Geometry: final body of the model. Coordinates: model frame, mm. Face numbers are marked on the shaded views. A direction names the side the tool comes from. Coordinates: 2 decimals unless noted, no trailing zeros. Order: outer loops, then holes, each group sorted by start corner. A loop starts at its lowest first (then second) coordinate and runs counter-clockwise, first axis right, second up. Notation, with made-up numbers: (-3.75, -26.75) - (28.25, -26.75) arc R11 cw to (28.25, -7.75) - close; hole circle Ø4 at (21.25, 23). An arc over 180 degrees is marked (long way). Use a Markdown table: item, result. Add a question column.
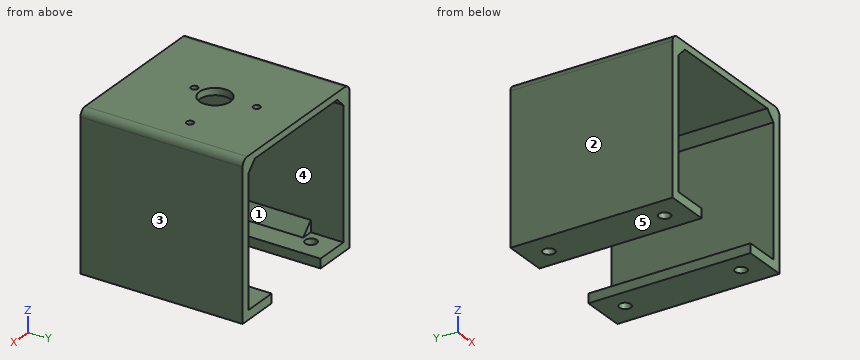
```python
from build123d import *

# Parameters (mm, degrees)
SKETCH1_W                = 70
SKETCH1_H                = 70
BOSS_EXTRUDE2_DEPTH      = 3
SKETCH2_R                = 6.75
SKETCH2_R_2              = 1.5
CUT_EXTRUDE1_DEPTH       = 4
SKETCH3_W                = 64
SKETCH3_H                = 70
BOSS_EXTRUDE3_DEPTH      = 4
SKETCH4_W                = 64
SKETCH4_H                = 70
BOSS_EXTRUDE4_DEPTH      = 4
SKETCH5_W                = 15
SKETCH5_H                = 70
BOSS_EXTRUDE5_DEPTH      = 4
SKETCH6_R                = 2.5
CUT_EXTRUDE2_DEPTH       = 4
BOSS_EXTRUDE6_DEPTH      = 70
BOSS_EXTRUDE7_DEPTH      = 20
BOSS_EXTRUDE7_DEPTH_BACK = 19
FILLET1_R                = 3


with BuildPart() as part:
    # Sketch1 → Boss-Extrude2 (new body)
    with BuildSketch(Plane.XY):
        with Locations((-9.605752423, -0.918004132)):
            Rectangle(SKETCH1_W, SKETCH1_H)
    extrude(amount=BOSS_EXTRUDE2_DEPTH)

    # Sketch2 → Cut-Extrude1 (cut)
    with BuildSketch(Plane.XY.offset(3)):
        with Locations((-9.605752423, -0.918004132)):
            Circle(SKETCH2_R)
        with Locations((-11.293574597, 16.005389627)):
            Circle(SKETCH2_R_2)
        with Locations((11.956425403, 2.581995868)):
            Circle(SKETCH2_R_2)
        with Locations((-11.293574597, -10.84139789)):
            Circle(SKETCH2_R_2)
    extrude(amount=-CUT_EXTRUDE1_DEPTH, mode=Mode.SUBTRACT)

    # Sketch3 → Boss-Extrude3 (add)
    with BuildSketch(Plane(origin=(25.394247577, 0, 0), x_dir=(0, 0, -1), z_dir=(1, 0, 0))):
        with Locations((32, -0.918004132)):
            Rectangle(SKETCH3_W, SKETCH3_H)
    extrude(amount=-BOSS_EXTRUDE3_DEPTH)

    # Sketch4 → Boss-Extrude4 (add)
    with BuildSketch(Plane.ZY.offset(44.605752423)):
        with Locations((-32, -0.918004132)):
            Rectangle(SKETCH4_W, SKETCH4_H)
    extrude(amount=-BOSS_EXTRUDE4_DEPTH)

    # Sketch5 → Boss-Extrude5 (add)
    with BuildSketch(Plane(origin=(0, 0, -64), x_dir=(-1, 0, 0), z_dir=(0, 0, -1))):
        with Locations((-13.894247577, -0.918004132)):
            Rectangle(SKETCH5_W, SKETCH5_H)
        with Locations((33.105752423, -0.918004132)):
            Rectangle(SKETCH5_W, SKETCH5_H)
    extrude(amount=-BOSS_EXTRUDE5_DEPTH)

    # Sketch6 → Cut-Extrude2 (cut)
    with BuildSketch(Plane(origin=(0, 0, -64), x_dir=(-1, 0, 0), z_dir=(0, 0, -1))):
        with Locations((-15.394247577, 24.081995868)):
            Circle(SKETCH6_R)
        with Locations((-15.394247577, -25.918004132)):
            Circle(SKETCH6_R)
        with Locations((34.605752423, 24.081995868)):
            Circle(SKETCH6_R)
        with Locations((34.605752423, -25.918004132)):
            Circle(SKETCH6_R)
    extrude(amount=-CUT_EXTRUDE2_DEPTH, mode=Mode.SUBTRACT)

    # Sketch7 → Boss-Extrude6 (add)
    with BuildSketch(Plane(origin=(0, 34.081995868, 0), x_dir=(1, 0, 0), z_dir=(0, 1, 0))):
        Polygon((-40.605752423, 0), (-40.605752423, 4), (-36.605752423, 0), align=None)
        Polygon((21.394247577, 0), (21.394247577, 4), (17.394247577, 0), align=None)
    extrude(amount=-BOSS_EXTRUDE6_DEPTH)

    # Sketch8 → Boss-Extrude7 (add, two sides: drawn at the far end of the back side and taken through both)
    with BuildSketch(Plane(origin=(0, 0, 0), x_dir=(1, 0, 0), z_dir=(0, 1, 0)).offset(-BOSS_EXTRUDE7_DEPTH_BACK)):
        Polygon((-40.605752423, 60), (-35.605752423, 60), (-40.605752423, 55), align=None)
        Polygon((21.394247577, 60), (16.394247577, 60), (21.394247577, 55), align=None)
    extrude(amount=BOSS_EXTRUDE7_DEPTH + BOSS_EXTRUDE7_DEPTH_BACK)

    # Fillet1
    fillet1_edges = [part.edges().sort_by_distance(p)[0] for p in [
        (25.394247577, -0.918004132, 3),
        (-44.605752423, -0.918004132, 3),
    ]]
    fillet(fillet1_edges, radius=FILLET1_R)


solid = part.part
```
1) Draft query along Z for the marked faces 3, 4 and 5. Return one class per face: pulls with the +Z half, pulls with the -Z half, needs draft (parallel to the pull), parting line crosses it, or undercut.
2) Section D-D (y = -3). Return loops of the section in (x, z).
3) Section C-C (z = -43.5). Return loops of the section in (x, y).
4) Section B-B (y = 10.5). Return loops of the section in (x, z).
5) Ray query, line 1 along X through (y, z) = (3, -16); line 2 along Z through (x, y) = (-28, 21); line 3 along Z through (x, y) = (-34.5, 25.5). Return the intervals inside material, ascending.
6) Section A-A (x = -30). Return loops of the section in (y, z), then the cut area to 3 significant figures.
7) Set-up query: the marked faces 1 and 2. Return all of +Z, -Z, +X, -X, +Y, -Y with unobstructed straight access to the full face (end or side cutting, diameter ignored); none if empty.
8) Pin query (flat end, axial travel): pin 1 (11 mm diameter, centred on x = -9.61, y = -0.92, fed in from -Z); pin 2 (6 mm diameter, centred on x = -34.61, y = -25.92, fed in from -Z); pin 3 (4 mm diameter, centred on x = -11.29, y = -10.84, fed in from -Z); pin 4 (2.5 mm diameter, centred on x = 20, z = -56.5, fed in from -Y). Return the tip coordinate at first contact, or that it passes through.
Values follow:
| question | item | result |
|---|---|---|
| 1 | face 3 | needs draft |
| 1 | face 4 | undercut |
| 1 | face 5 | pulls with the -Z half |
| 2 | outline | (-44.61, -64) - (-25.61, -64) - (-25.61, -60) - (-35.61, -60) - (-40.61, -55) - (-40.61, -4) - (-36.61, 0) - (-16.03, 0) - (-16.03, 3) - (-41.61, 3) arc R3 ccw to (-44.61, 0) - close; (-3.18, 0) - (17.39, 0) - (21.39, -4) - (21.39, -55) - (16.39, -60) - (6.39, -60) - (6.39, -64) - (25.39, -64) - (25.39, 0) arc R3 ccw to (22.39, 3) - (-3.18, 3) - close |
| 3 | outline | (-44.61, -35.92) - (-40.61, -35.92) - (-40.61, 34.08) - (-44.61, 34.08) - close; (21.39, -35.92) - (25.39, -35.92) - (25.39, 34.08) - (21.39, 34.08) - close |
| 4 | outline | (-44.61, -64) - (-25.61, -64) - (-25.61, -60) - (-35.61, -60) - (-40.61, -55) - (-40.61, -4) - (-36.61, 0) - (17.39, 0) - (21.39, -4) - (21.39, -55) - (16.39, -60) - (6.39, -60) - (6.39, -64) - (25.39, -64) - (25.39, 0) arc R3 ccw to (22.39, 3) - (-41.61, 3) arc R3 ccw to (-44.61, 0) - close |
| 5 | line 1 | x = -44.61 to -40.61, 21.39 to 25.39 |
| 5 | line 2 | z = -64 to -60, 0 to 3 |
| 5 | line 3 | z = 0 to 3 |
| 6 | outline | (-35.92, -64) - (34.08, -64) - (34.08, -60) - (-35.92, -60) - close; (-35.92, 0) - (34.08, 0) - (34.08, 3) - (-35.92, 3) - close |
| 6 | area | 490 mm² |
| 7 | face 1 | +Y, -Y |
| 7 | face 2 | +Z, -Z, -X, +Y, -Y |
| 8 | pin 1 | passes through |
| 8 | pin 2 | stops at z = -64 |
| 8 | pin 3 | stops at z = 0 |
| 8 | pin 4 | stops at y = -19 |
